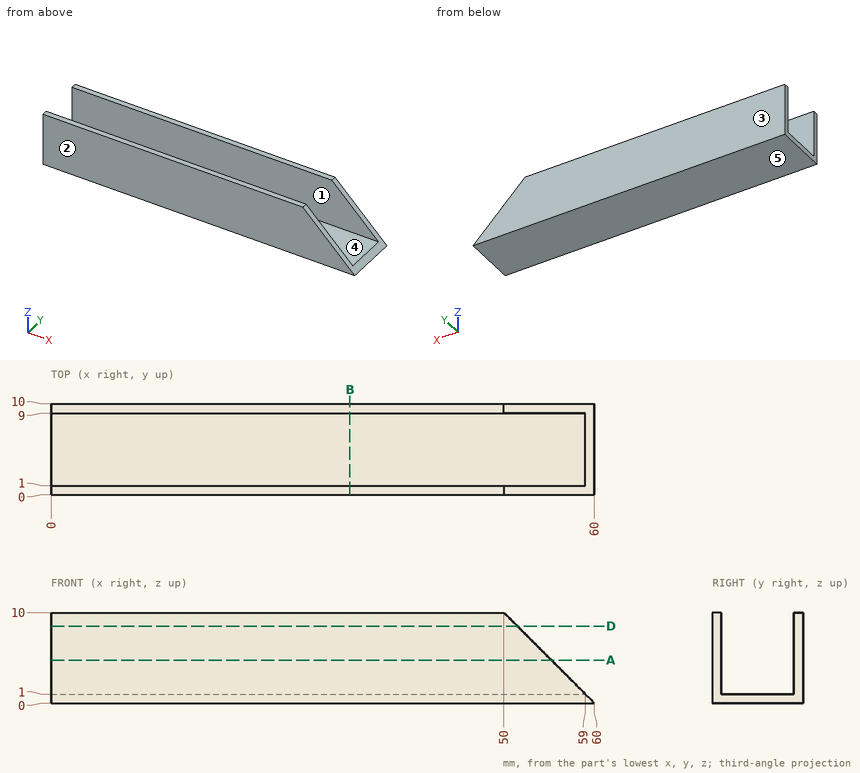
Input: dimensioned drawing with shaded views. Units: mm. Origin: part minimum x, y, z. A direction names the side the tool comes from. Give positions to 0.01 mm unless a question says otherwise; leave off trailing zeros. Order: outer loops, then holes, each group sorted by start corner. A loop starts at its lowest first (then second) coordinate and runs counter-clockwise, first axis right, second up. Notation, with made-up numbers: (45.5, 23.5) -> (66.5, 23.5) arc R15 ccw to (66.5, 29.5) -> close; hole circle Ø3 at (78.5, 36.5). An arc over 180 degrees is marked (long way). Write item = value, one per line.
Item 1: Mould query, pull axis Y, two halves, no side actions, for the marked faces 3, 4 and 5. Classes: +Y half, -Y half, draft (parallel to the pull), parting line (faces both ways), or undercut.
Check result:
face_3 = +Y half
face_4 = undercut
face_5 = draft
Item 2: Section query D-D (z = 8.5). Output: boundary loops of the cut face in (x, y), then the cut area to 3 significant figures.
Check result:
outline = (0, 0) -> (51.5, 0) -> (51.5, 1) -> (0, 1) -> close; (0, 9) -> (51.5, 9) -> (51.5, 10) -> (0, 10) -> close
area = 103 mm²
Item 3: Contact query for a flat-ended pin moving along its axis: pin 1 (4 mm diameter, centred on x = 41, y = 5, fed in from +Z). Output: stop coordinate, or through.
Check result:
pin_1 = 1
Item 4: Section query B-B (x = 33). Output: boundary loops of the cut face in (y, z).
Check result:
outline = (0, 0) -> (10, 0) -> (10, 10) -> (9, 10) -> (9, 1) -> (1, 1) -> (1, 10) -> (0, 10) -> close
Item 5: Set-up query: the marked faces 1 and 2. Return all of +Z, -Z, +X, -X, +Y, -Y with unobstructed straight access to the full face (end or side cutting, diameter ignored); none if empty.
Check result:
face_1 = +Z, +X, -X
face_2 = +Z, -Z, +X, -X, -Y
Item 6: Section query A-A (z = 4.75). Output: boundary loops of the cut face in (x, y).
Check result:
outline = (0, 0) -> (55.25, 0) -> (55.25, 1) -> (0, 1) -> close; (0, 9) -> (55.25, 9) -> (55.25, 10) -> (0, 10) -> close
Item 7: Ray query, probe 1 along Y at (x, z) = (54.5, 3); probe 2 along Z at (x, y) = (14.5, 8.5); probe 3 along X at (y, z) = (9.5, 7). Return the intervals inside material, ascending.
Check result:
probe_1 = 0 to 1, 9 to 10
probe_2 = 0 to 1
probe_3 = 0 to 53
